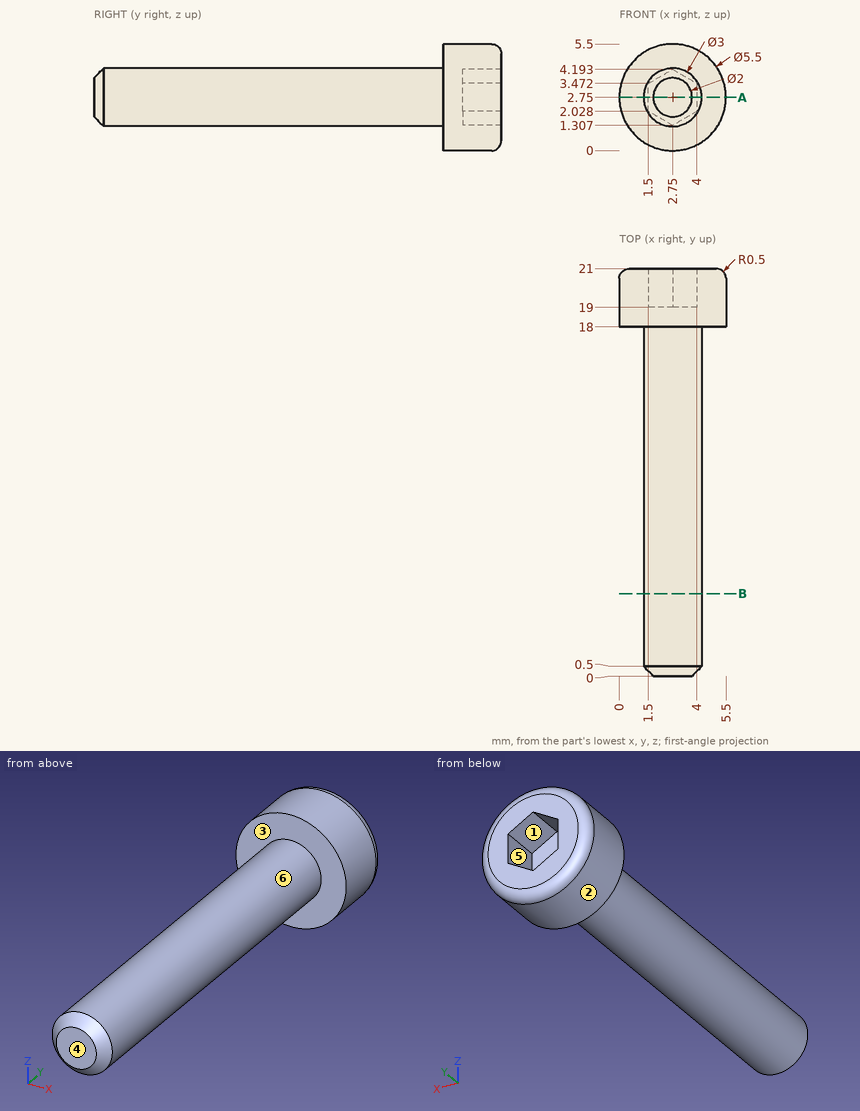
Part print with two shaded views. Sizes in mm from the minimum x, y, z corner. A direction names the side the tool comes from. Round coordinates to 2 decimals unless told otherwise and drop trailing zeros. Loops run counter-clockwise (first coordinate to the right, second up) from the corner with the lowest first, then second, coordinate; pieces in that order, holes last.
1. Slice it at B-B (y = 4.25). Give the cut face in (x, z).
Solutions:
outline: circle Ø3 at (2.75, 2.75)
2. Flat gauge pins, fed straight in: pin 1 (2 mm diameter, centred on x = 2, z = 1, fed in from -Y); pin 2 (1 mm diameter, centred on y = 18, z = 0.5, fed in from +X); pin 3 (0.8 mm diameter, centred on x = 2.5, z = 2, fed in from +Y). Where does each tip first touch, or does it go through?
Solutions:
pin 1: stops at y = 0
pin 2: stops at x = 4.87
pin 3: stops at y = 19
3. 3-axis set-ups, long thin cutter, end or side, ignore diameter. For the marked faces 4, 5 and 6: which of +Z, -Z, +X, -X, +Y, -Y reach the whole face in a straight line?
Solutions:
face 4: +Z, -Z, +X, -X, -Y
face 5: +Y
face 6: -Y
4. Two-plate mould, pull along Z, no slides. Class the marked faces 1, 2 and 3: pulls with the +Z half, pulls with the -Z half, needs draft (parallel to the pull), parting line crosses it, or undercut.
Solutions:
face 1: undercut
face 2: parting line crosses it
face 3: needs draft
5. Slice it at A-A (z = 2.75). Give the cut face in (x, y).
Solutions:
outline: (0, 18) - (1.25, 18) - (1.25, 0.5) - (1.75, 0) - (3.75, 0) - (4.25, 0.5) - (4.25, 18) - (5.5, 18) - (5.5, 20.5) arc R0.5 ccw to (5, 21) - (4, 21) - (4, 19) - (1.5, 19) - (1.5, 21) - (0.5, 21) arc R0.5 ccw to (0, 20.5) - close
6. Drill centre lines: line 1 along Y through (x, z) = (2.15, 3.25); line 2 along Y through (x, z) = (0.5, 2.7); line 3 along X through (y, z) = (7.5, 2.85). Where is each one in solid material? Low to high.
Solutions:
line 1: y = 0 to 19
line 2: y = 18 to 21
line 3: x = 1.25 to 4.25
